Could you check a few things on this drawing? It's one solid part, dimensions in mm from its lowest x, y, z. A direction names the side the tool comes from. Give positions to 0.01 mm unless a question says otherwise; leave off trailing zeros. Order: outer loops, then holes, each group sorted by start corner. A loop starts at its lowest first (then second) coordinate and runs counter-clockwise, first axis right, second up.
(1) Imagine slicing it at C-C, the plane z = 17. Write out the boundary of the cut face in (x, y), then the cut area to 3 significant figures.
(2) On a 3-axis mill with a long thin cutter (end or side, diameter ignored), from which of +Z, -Z, +X, -X, +Y, -Y can I reach the whole of each face in a straight line? I mean the marked faces 1 and 2. Say none if no direction works.
(3) Will these pins go through, and if not, where does the flat tip stop? pin 1 (5 mm diameter, centred on y = 67.5, z = 35.5, fed in from -X) (3 decimals); pin 2 (10 mm diameter, centred on x = 52.5, z = 22.5, fed in from +Y); pin 3 (8 mm diameter, centred on y = 30.5, z = 12.5, fed in from +X).
(4) If we mould it in two halves opening along Y, with no side actions, what happens to the marked faces 3, 4 and 5? For each: released by +Y, released by -Y, zero draft, split by the parting line, or undercut.
(5) Imagine slicing it at A-A, the plane x = 40. Write out the boundary of the cut face in (y, z) (3 decimals), then the cut area to 3 significant figures.
(6) If I drill on probe 1 along X at (y, z) = (40, 11); probe 2 along Z at (x, y) = (59, 74.5); probe 3 along X at (y, z) = (33.5, 28), over which ranges is the centre line in solid material (lowest first)?
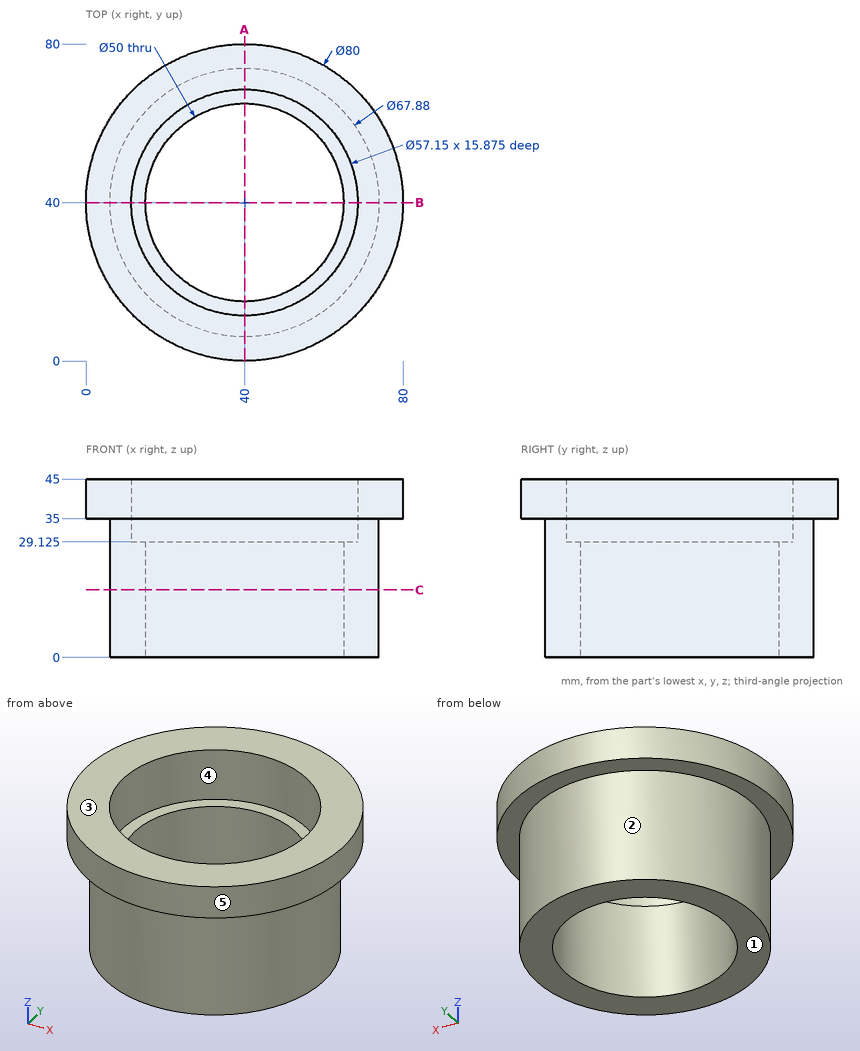
Answer block:
1. outline: circle Ø67.88 at (40, 40); hole circle Ø50 at (40, 40)
1. area: 1,660 mm2
2. face 1: -Z, +X, -X, +Y, -Y
2. face 2: -Z
3. pin 1: stops at x = 8.775
3. pin 2: stops at y = 73.1
3. pin 3: stops at x = 73.49
4. face 3: zero draft
4. face 4: undercut
4. face 5: split by the parting line
5. outline: (0, 35) - (6.06, 35) - (6.06, 0) - (15, 0) - (15, 29.125) - (11.425, 29.125) - (11.425, 45) - (0, 45) - close; (65, 0) - (73.94, 0) - (73.94, 35) - (80, 35) - (80, 45) - (68.575, 45) - (68.575, 29.125) - (65, 29.125) - close
5. area: 812 mm2
6. probe 1: x = 6.06 to 15, 65 to 73.94
6. probe 2: z = 35 to 45
6. probe 3: x = 6.69 to 15.86, 64.14 to 73.31
